The listing builds one solid part. Answer for the finished solid, in the listing's coordinates (mm). A direction names the side the tool comes from. Coordinates: 2 decimals unless noted, no trailing zeros. Order: outer loops, then holes, each group sorted by start corner. A loop starts at its lowest first (then second) coordinate and runs counter-clockwise, first axis right, second up. Notation, with made-up numbers: (80.25, 33) -> (104.25, 33) arc R14 ccw to (104.25, 38) -> close; hole circle Ø5 at (13.25, 89). An arc over 180 degrees is marked (long way). Write item = value, one per line.
Autodesk Inventor part; units mm, degrees
ref_plane "YZ Plane" through (0, 0, 0) normal (1, 0, 0) x (0, 1, 0)
ref_plane "XZ Plane" through (0, 0, 0) normal (0, 1, 0) x (-1, 0, 0)
ref_plane "XY Plane" through (0, 0, 0) normal (0, 0, 1) x (1, 0, 0)
sketch "Sketch1" plane through (0, 0, 0) normal (0, 0, 1) x (1, 0, 0)
  line L0 (-74, 14.75) -> (54, 14.75) construction
  line L1 (-89.2201, 0) -> (135.4294, 0) construction
  circle A0 centre (-74, 14.75) radius 1.525
  circle A1 centre (-32, 14.75) radius 1.525
  circle A2 centre (54, 14.75) radius 1.525
  line L2 (-77.5, 0.7411) -> (-77.5, 20.25)
  line L3 (-77.5, 20.25) -> (77.5, 20.25)
  line L4 (77.5, 20.25) -> (77.5, 0)
  line L5 (-74, -14.75) -> (54, -14.75) construction
  circle A3 centre (-74, -14.75) radius 1.525
  circle A4 centre (-32, -14.75) radius 1.525
  circle A5 centre (54, -14.75) radius 1.525
  line L6 (-77.5, -0.7411) -> (-77.5, -20.25)
  line L7 (-77.5, -20.25) -> (77.5, -20.25)
  line L8 (77.5, -20.25) -> (77.5, 0)
  line L9 (-77.5, 0.7411) -> (-77.5, -0.7411)
  point P0 (0, 0)
  point P1 (0, 0)
  dimension "d2" = 3.05
  dimension "d3" = 3.05
  dimension "d4" = 3.05
  dimension "d6" = 42
  dimension "d7" = 86
  dimension "d127" = 20.25
  dimension "d129" = 155
  dimension "d130" = 77.5
  dimension "d131" = 3.5
extrude "Extrusion1" add sketch "Sketch1" along normal blind 1
sketch "Sketch5" plane through (0, 0, 1) normal (0, 0, 1) x (1, 0, 0)
  line L0 (-59.5, -18) -> (-65.5, -20.25)
  line L1 (-77.5, -11) -> (-65.5, -11)
  line L2 (0, 40.5196) -> (0, -40.5196)
  line L3 (-109.7892, 0) -> (116.2355, 0)
  line L4 (-60.5, -6) -> (-60.5, 0)
  arc A0 (-65.5, -11) -> (-60.5, -6) centre (-65.5, -6) ccw
  circle A1 centre (54, -14.75) radius 1.525
  arc A2 (52.701, -18) -> (57.1503, -16.275) centre (54, -14.75) ccw
  line L5 (52.701, -18) -> (-59.5, -18)
  line L6 (57.1503, -16.275) -> (77.5, -12.6734)
  arc A3 (57.1503, -16.275) -> (52.701, -18) centre (54, -14.75) ccw construction
  line L7 (49, -11) -> (40, -11)
  line L8 (36.5, -7.5) -> (36.5, 0)
  line L9 (52.5, 0) -> (52.5, -7.5)
  line L10 (-42, -8) -> (-50, -8)
  line L11 (-53.5, -4.5) -> (-53.5, 0)
  line L12 (-38.5, 0) -> (-38.5, -4.5)
  line L13 (-30.5, 0) -> (-30.5, -6.5)
  line L14 (-33.5, -6.5) -> (-33.5, 0)
  arc A4 (-33.5, -6.5) -> (-30.5, -6.5) centre (-32, -6.5) ccw
  line L15 (-9.5, 0) -> (-9.5, -4.5)
  line L16 (-13, -8) -> (-21, -8)
  line L17 (-24.5, -4.5) -> (-24.5, 0)
  line L18 (10, -8) -> (2, -8)
  line L19 (-1.5, -4.5) -> (-1.5, 0)
  line L20 (13.5, 0) -> (13.5, -4.5)
  circle A5 centre (-32, -14.75) radius 1.525 construction
  line L21 (-32, -14.75) -> (15.7139, -14.75) construction
  circle A6 centre (-32, 14.75) radius 1.525 construction
  line L22 (-32, 14.75) -> (13.5, 14.75) construction
  line L23 (12, -28.9426) -> (12, 23.2337) construction
  line L24 (0, -27.2548) -> (0, 23.7474) construction
  line L25 (-11, -24.7597) -> (-11, 23.7474) construction
  line L26 (-23, -24.7597) -> (-23, 23.7474) construction
  line L27 (12, -14.75) -> (0, -14.75) construction
  line L28 (12, -13.25) -> (0, -13.25)
  line L29 (0, -16.25) -> (12, -16.25)
  arc A7 (12, -16.25) -> (12, -13.25) centre (12, -14.75) ccw
  arc A8 (0, -13.25) -> (0, -16.25) centre (0, -14.75) ccw
  line L30 (-11, -14.75) -> (-23, -14.75) construction
  line L31 (-11, -13.25) -> (-23, -13.25)
  line L32 (-23, -16.25) -> (-11, -16.25)
  arc A9 (-11, -16.25) -> (-11, -13.25) centre (-11, -14.75) ccw
  arc A10 (-23, -13.25) -> (-23, -16.25) centre (-23, -14.75) ccw
  arc A11 (49, -11) -> (52.5, -7.5) centre (49, -7.5) ccw
  arc A12 (36.5, -7.5) -> (40, -11) centre (40, -7.5) ccw
  arc A13 (10, -8) -> (13.5, -4.5) centre (10, -4.5) ccw
  arc A14 (-1.5, -4.5) -> (2, -8) centre (2, -4.5) ccw
  arc A15 (-13, -8) -> (-9.5, -4.5) centre (-13, -4.5) ccw
  arc A16 (-24.5, -4.5) -> (-21, -8) centre (-21, -4.5) ccw
  arc A17 (-42, -8) -> (-38.5, -4.5) centre (-42, -4.5) ccw
  arc A18 (-53.5, -4.5) -> (-50, -8) centre (-50, -4.5) ccw
  line L33 (-59.5, 18) -> (-65.5, 20.25)
  line L34 (-77.5, 11) -> (-65.5, 11)
  line L35 (-60.5, 6) -> (-60.5, 0)
  arc A19 (-60.5, 6) -> (-65.5, 11) centre (-65.5, 6) ccw
  circle A20 centre (54, 14.75) radius 1.525
  arc A21 (57.1503, 16.275) -> (52.701, 18) centre (54, 14.75) ccw
  line L36 (52.701, 18) -> (-59.5, 18)
  line L37 (57.1503, 16.275) -> (77.5, 12.6734)
  arc A22 (52.701, 18) -> (57.1503, 16.275) centre (54, 14.75) ccw construction
  line L38 (49, 11) -> (40, 11)
  line L39 (36.5, 7.5) -> (36.5, 0)
  line L40 (52.5, 0) -> (52.5, 7.5)
  line L41 (-42, 8) -> (-50, 8)
  line L42 (-53.5, 4.5) -> (-53.5, 0)
  line L43 (-38.5, 0) -> (-38.5, 4.5)
  line L44 (-30.5, 0) -> (-30.5, 6.5)
  line L45 (-33.5, 6.5) -> (-33.5, 0)
  arc A23 (-30.5, 6.5) -> (-33.5, 6.5) centre (-32, 6.5) ccw
  line L46 (-9.5, 0) -> (-9.5, 4.5)
  line L47 (-13, 8) -> (-21, 8)
  line L48 (-24.5, 4.5) -> (-24.5, 0)
  line L49 (10, 8) -> (2, 8)
  line L50 (-1.5, 4.5) -> (-1.5, 0)
  line L51 (13.5, 0) -> (13.5, 4.5)
  circle A24 centre (-32, 14.75) radius 1.525 construction
  line L52 (-32, 14.75) -> (15.7139, 14.75) construction
  line L53 (12, 14.75) -> (0, 14.75) construction
  line L54 (12, 13.25) -> (0, 13.25)
  line L55 (0, 16.25) -> (12, 16.25)
  arc A25 (12, 13.25) -> (12, 16.25) centre (12, 14.75) ccw
  arc A26 (0, 16.25) -> (0, 13.25) centre (0, 14.75) ccw
  line L56 (-11, 14.75) -> (-23, 14.75) construction
  line L57 (-11, 13.25) -> (-23, 13.25)
  line L58 (-23, 16.25) -> (-11, 16.25)
  arc A27 (-11, 13.25) -> (-11, 16.25) centre (-11, 14.75) ccw
  arc A28 (-23, 16.25) -> (-23, 13.25) centre (-23, 14.75) ccw
  arc A29 (52.5, 7.5) -> (49, 11) centre (49, 7.5) ccw
  arc A30 (40, 11) -> (36.5, 7.5) centre (40, 7.5) ccw
  arc A31 (13.5, 4.5) -> (10, 8) centre (10, 4.5) ccw
  arc A32 (2, 8) -> (-1.5, 4.5) centre (2, 4.5) ccw
  arc A33 (-9.5, 4.5) -> (-13, 8) centre (-13, 4.5) ccw
  arc A34 (-21, 8) -> (-24.5, 4.5) centre (-21, 4.5) ccw
  arc A35 (-38.5, 4.5) -> (-42, 8) centre (-42, 4.5) ccw
  arc A36 (-50, 8) -> (-53.5, 4.5) centre (-50, 4.5) ccw
  line L59 (77.5, -12.6734) -> (82.2803, -14.75)
  line L60 (82.2803, -14.75) -> (77.5, -28.9426)
  line L61 (77.5, -28.9426) -> (-65.5, -24.3901)
  line L62 (-65.5, -24.3901) -> (-65.5, -20.25)
  line L63 (77.5, 12.6734) -> (83.9462, 22.4701)
  line L64 (83.9462, 22.4701) -> (-65.5, 21.6624)
  line L65 (-65.5, 21.6624) -> (-65.5, 20.25)
  line L66 (-77.5, -11) -> (-77.5, 11)
  point P0 (0, 0)
  point P1 (-77.5, -20.25)
  point P2 (-77.5, 20.25)
  point P3 (52.5, -11)
  point P4 (36.5, -11)
  point P5 (-38.5, -8)
  point P6 (-53.5, -8)
  point P7 (-9.5, -8)
  point P8 (-24.5, -8)
  point P9 (-1.5, -8)
  point P10 (6, -14.75)
  point P11 (-17, -14.75)
  point P12 (52.5, 11)
  point P13 (36.5, 11)
  point P14 (-38.5, 8)
  point P15 (-53.5, 8)
  point P16 (-9.5, 8)
  point P17 (-24.5, 8)
  point P18 (-1.5, 8)
  point P19 (12, 28.9426)
  point P20 (0, 27.2548)
  point P21 (-11, 24.7597)
  point P22 (-23, 24.7597)
  point P23 (6, 14.75)
  point P24 (-17, 14.75)
  dimension "d133" = 12
  dimension "d135" = 11
  dimension "d137" = 5
  dimension "d138" = 7
  dimension "d139" = 97
  dimension "d140" = 16
  dimension "d141" = 8
  dimension "d142" = 7
  dimension "d143" = 15
  dimension "d144" = 3
  dimension "d147" = 6.5
  dimension "d148" = 15
  dimension "d149" = 8
  dimension "d150" = 36
  dimension "d151" = 15
  dimension "d152" = 8
  dimension "d153" = 59
  dimension "d154" = 27
  dimension "d155" = 6.5
  dimension "d156" = 1.5
  dimension "d157" = 1.5
  dimension "d158" = 1.5
  dimension "d159" = 1.5
  dimension "d161" = 3.5
extrude "Extrusion5" cut sketch "Sketch5" against normal through all contours L5 L2 L61 L62 L0 | L4 A0 L1 L66 L3 | L3 L66 L34 A19 L35 | L12 A17 L10 A18 L11 L3 | L3 L42 A36 L41 A35 L43 | L13 A4 L14 L3 | L3 L45 A23 L44 | L15 A15 L16 A16 L17 L3 | L3 L48 A34 L47 A33 L46 | L36 L33 L65 L64 L2 | L2 L64 L63 L37 A21 L36 | A26 L2 | L2 L55 A25 L54 | L39 A30 L38 A29 L40 L3 | L3 L9 A11 L7 A12 L8 | A14 L19 L3 L2 | L2 L3 L20 A13 L18 A14 | A8 L2 | L2 L28 A7 L29 | L5 A2 L6 L59 L60 L61 L2 | L3 L50 A32 L2 | L2 A32 L49 A31 L51 L3 | A9 L32 A10 L31 | L57 A28 L58 A27
equation "\"d3\" = d2"
equation "\"d4\" = d2"
properties part number "Top Plate" material "CFRP"
Q1. Section C-C, the plane y = -2 is taken. Give the vertices of the cut face in (x, z).
The answers:
outline = (-60.5, 0) -> (-53.5, 0) -> (-53.5, 1) -> (-60.5, 1) -> close; (-38.5, 0) -> (-33.5, 0) -> (-33.5, 1) -> (-38.5, 1) -> close; (-30.5, 0) -> (-24.5, 0) -> (-24.5, 1) -> (-30.5, 1) -> close; (-9.5, 0) -> (-1.5, 0) -> (-1.5, 1) -> (-9.5, 1) -> close; (13.5, 0) -> (36.5, 0) -> (36.5, 1) -> (13.5, 1) -> close; (52.5, 0) -> (77.5, 0) -> (77.5, 1) -> (52.5, 1) -> close
Q2. A tool of negligible diameter and unlimited length cuts with its end or side. For faces 1 (the face through (-1, -9, 0)), 2 (the face through (-52.45, 7, 0.51)), from which of +Z, -Z, +X, -X, +Y, -Y can it reach the whole face along a straight path? Write none if from no direction.
The answers:
face_1 = -Z, +X, -X, +Y, -Y
face_2 = +Z, -Z
Q3. Section B-B, the plane x = -74 is taken. Give the vertices of the cut face in (y, z) (3 decimals).
The answers:
outline = (-20.25, 0) -> (-16.275, 0) -> (-16.275, 1) -> (-20.25, 1) -> close; (-13.225, 0) -> (-11, 0) -> (-11, 1) -> (-13.225, 1) -> close; (11, 0) -> (13.225, 0) -> (13.225, 1) -> (11, 1) -> close; (16.275, 0) -> (20.25, 0) -> (20.25, 1) -> (16.275, 1) -> close
Q4. Section D-D, the plane x = 54 is taken. Give the vertices of the cut face in (y, z) (3 decimals).
The answers:
outline = (-18.25, 0) -> (-16.275, 0) -> (-16.275, 1) -> (-18.25, 1) -> close; (-13.225, 0) -> (13.225, 0) -> (13.225, 1) -> (-13.225, 1) -> close; (16.275, 0) -> (18.25, 0) -> (18.25, 1) -> (16.275, 1) -> close
Q5. Each of these flat-tipped pins is pushed along its axis until it touches: pin 1 Ø0.5 at (x, z) = (-18, 0.5) entering from +Y; pin 2 Ø0.5 at (y, z) = (-0.5, 0.5) entering from -X. Where does it stop, or does it pass through?
The answers:
pin_1 = 18
pin_2 = -60.5
Q6. Find the intervals of material crossed by line 1 along Y through (x, z) = (-74, 0.75) (3 decimals); line 2 along Y through (x, z) = (54, 0.25) (3 decimals); line 3 along Y through (x, z) = (-32, 0.45) (3 decimals), in increasing order.
The answers:
line_1 = -20.25 to -16.275, -13.225 to -11, 11 to 13.225, 16.275 to 20.25
line_2 = -18.25 to -16.275, -13.225 to 13.225, 16.275 to 18.25
line_3 = -18 to -16.275, -13.225 to -8, 8 to 13.225, 16.275 to 18
Q7. Section A-A, the plane x = -44.5 is taken. Give the vertices of the cut face in (y, z), plus the area to 3 significant figures.
The answers:
outline = (-18, 0) -> (-8, 0) -> (-8, 1) -> (-18, 1) -> close; (8, 0) -> (18, 0) -> (18, 1) -> (8, 1) -> close
area = 20.0 mm2
Q8. The mould has two halves that part along X. Classify faces 3 (the face through (67.18, 14.5, 0.51)), 4 (the face through (-62, -9.57, 0.51)), 5 (the face through (-1, -9, 1)), 6 (the face through (-39.55, -7, 0.51)): released by +X, released by -X, zero draft, split by the parting line, or undercut.
The answers:
face_3 = released by +X
face_4 = released by -X
face_5 = zero draft
face_6 = undercut
